Could you check a few things on this model? Use its own coordinates, in mm. A direction names the side the tool comes from. Coordinates: 2 decimals unless noted, no trailing zeros. Loops run counter-clockwise (first coordinate to the right, second up) from the corner with the lowest first, then second, coordinate; pieces in that order, holes last. Notation, with made-up numbers: (-34, 0.25) - (-8, 0.25) arc R6 ccw to (-8, 5.25) - close; hole circle Ø10 at (31, -12.75). An arc over 180 degrees is marked (long way). Put each result on its own line as item: value. Start each with the question number.
```python
from build123d import *

# Parameters (mm, degrees)
SKETCH_1_R          = 5
EXTRUDE_1_DEPTH     = 5
SKETCH_3_R          = 3
EXTRUDE_2_DEPTH     = 2
EXTRUDE_3_DEPTH     = 3
SKETCH_5_R          = 2.5
CUT_EXTRUDE_2_DEPTH = 6
CUT_EXTRUDE_1_DEPTH = 3


with BuildPart() as part:
    # 草图1 → 凸台-拉伸1 (new body)
    with BuildSketch(Plane(origin=(0, 0, 0), x_dir=(1, 0, 0), z_dir=(0, 1, 0))):
        with Locations(Location((0, 0, 0), (0, 0, 270))):
            Circle(SKETCH_1_R)
    extrude(amount=EXTRUDE_1_DEPTH)

    # 草图3 → 凸台-拉伸2 (add)
    with BuildSketch(Plane.XZ):
        with Locations(Location((0, 0, 0), (0, 0, 90))):
            Circle(SKETCH_3_R)
    extrude(amount=EXTRUDE_2_DEPTH)

    # 草图4 → 凸台-拉伸3 (add)
    with BuildSketch(Plane.XZ.offset(2)):
        Polygon((4.993690859, 5.00630119), (-5.00630119, 4.993690859), (-4.993690859, -5.00630119), (5.00630119, -4.993690859), align=None)
    extrude(amount=EXTRUDE_3_DEPTH)

    # 草图5 → 切除-拉伸2 (cut)
    with BuildSketch(Plane.XZ.offset(5)):
        with Locations(Location((0, 0, 0), (0, 0, 270))):
            Circle(SKETCH_5_R)
    extrude(amount=-CUT_EXTRUDE_2_DEPTH, mode=Mode.SUBTRACT)

    # 草图2 → 切除-拉伸1 (cut)
    with BuildSketch(Plane(origin=(0, 5, 0), x_dir=(1, 0, 0), z_dir=(0, 1, 0))):
        Polygon((-2.285405043, -1.130010526), (2.544224088, 0.1640847), (2.285405043, 1.130010526), (-2.544224088, -0.1640847), align=None)
    extrude(amount=-CUT_EXTRUDE_1_DEPTH, mode=Mode.SUBTRACT)


solid = part.part
```
(1) If we mould it in two halves opening along Y, with no side actions, what happens to faces 1 (the flat face through (0, 2, 0)), 2 (the cylindrical face through (-4.88, 2.46, -1.08)), 3 (the flat face through (2.2, -2, 2.3))? For each: pulls with the +Y half, pulls with the -Y half, needs draft (parallel to the pull), parting line crosses it, or undercut.
(2) Which directions (+Z, -Z, +X, -X, +Y, -Y) give clear straight access to the entire face, cutting with the end or side of a thin tool? Please do faces 4 (the flat face through (-0.1, 3.52, -0.49)), 5 (the flat face through (0, 1, 0)), 6 (the cylindrical face through (-0.9, -0.99, 2.86)).
(3) I want a section at C-C on z = 0. List the corners of the cut face in (x, y) for me, and give its area (3 significant figures).
(4) For pin 1 Ø1 at (x, z) = (-2, 1) entering from -Y; pin 2 Ø5 at (y, z) = (1, 3) entering from -X; pin 3 Ø2.5 at (x, z) = (0, 1) entering from -Y; pin 4 Ø2 at (y, z) = (-3.5, 2.5) entering from +X, each with a flat end and sliding along its axis, tell me the tip position at first contact or that it passes through.
(5) I need wall thicknesses on L1, parallel to X at y = -3, z = 0; L2, parallel to Y at x = 3.75, z = -3.25; L3, parallel to X at y = -1.15, z = 0. Which ranges of each line are inside material? Lowest first, please. Write a range as [from, to].
(6) I want a section at A-A on y = -2.5. List the corners of the cut face in (x, z) for me.
(7) I want a section at B-B on z = 4. List the corners of the cut face in (x, y) for me.
(8) I want a section at D-D on x = 2. List the corners of the cut face in (y, z) for me.
Answer sheet:
1. face 1: pulls with the +Y half
1. face 2: needs draft
1. face 3: undercut
2. face 4: +Y
2. face 5: -Y
2. face 6: none
3. outline: (-5, -5) - (-2.5, -5) - (-2.5, 1) - (2.5, 1) - (2.5, -5) - (5, -5) - (5, -2) - (3, -2) - (3, 0) - (5, 0) - (5, 5) - (1.93, 5) - (1.93, 2) - (-1.93, 2) - (-1.93, 5) - (-5, 5) - (-5, 0) - (-3, 0) - (-3, -2) - (-5, -2) - close
3. area: 50.4 mm^2
4. pin 1: stops at y = -5
4. pin 2: stops at x = -4.97
4. pin 3: stops at y = 1
4. pin 4: stops at x = 5
5. L1: x = [-5, -2.5], [2.5, 5]
5. L2: y = [-5, -2], [0, 5]
5. L3: x = [-3, -2.5], [2.5, 3]
6. outline: (-5.01, 4.99) - (-4.99, -5.01) - (5.01, -4.99) - (4.99, 5.01) - close; hole circle Ø5 at (0, 0)
7. outline: (-5.01, -5) - (4.99, -5) - (4.99, -2) - (-5.01, -2) - close; (-3, 0) - (3, 0) - (3, 5) - (-3, 5) - close
8. outline: (-5, -5) - (-2, -5) - (-2, -2.24) - (0, -2.24) - (0, -4.58) - (5, -4.58) - (5, -1.05) - (2, -1.05) - (2, -0.02) - (5, -0.02) - (5, 4.58) - (0, 4.58) - (0, 2.24) - (-2, 2.24) - (-2, 5) - (-5, 5) - (-5, 1.5) - (1, 1.5) - (1, -1.5) - (-5, -1.5) - close
